```python
from build123d import *

# Parameters (mm, degrees)
BOSS_EXTRUDE1_DEPTH = 10
SKETCH2_R           = 3.829706391
CUT_EXTRUDE1_DEPTH  = 10
CIRPATTERN1_COUNT   = 7
CIRPATTERN1_ANGLE   = 198
CUT_EXTRUDE2_DEPTH  = 10
CIRPATTERN2_COUNT   = 5
CIRPATTERN2_ANGLE   = 60
FILLET1_R           = 3
FILLET2_R           = 1


with BuildPart() as part:
    # Sketch1 → Boss-Extrude1 (new body)
    with BuildSketch(Plane(origin=(0, 0, 0), x_dir=(1, 0, 0), z_dir=(0, 1, 0))):
        with BuildLine():
            Line((-45.667120744, 35.07764347), (41.365145602, 35.07764347))
            ThreePointArc((41.365145602, 35.07764347), (76.442789072, 0), (41.365145602, -35.07764347))
            Line((41.365145602, -35.07764347), (-45.667120744, -35.07764347))
            ThreePointArc((-45.667120744, -35.07764347), (-80.744764215, 0), (-45.667120744, 35.07764347))
        make_face()
    extrude(amount=BOSS_EXTRUDE1_DEPTH)

    # Sketch2 → Cut-Extrude1 (cut)
    with BuildSketch(Plane(origin=(0, 10, 0), x_dir=(1, 0, 0), z_dir=(0, 1, 0))):
        with Locations((0, 21.114814392)):
            Circle(SKETCH2_R)
    cut_extrude1 = extrude(amount=-CUT_EXTRUDE1_DEPTH, mode=Mode.SUBTRACT)

    # CirPattern1: Cut-Extrude1 ×7 about axis
    cirpattern1_axis = Axis((-2.160973251, 0, 0.098022779), (0, 1, 0))
    for i in range(1, CIRPATTERN1_COUNT):
        add(cut_extrude1.rotate(cirpattern1_axis, i * CIRPATTERN1_ANGLE / (CIRPATTERN1_COUNT - 1)), mode=Mode.SUBTRACT)

    # Sketch3 → Cut-Extrude2 (cut)
    with BuildSketch(Plane(origin=(0, 10, 0), x_dir=(1, 0, 0), z_dir=(0, 1, 0))):
        Polygon((36.992565085, 19.326531544), (35.239702282, 24.889438713), (31.298514755, 20.589961412), align=None)
    cut_extrude2 = extrude(amount=-CUT_EXTRUDE2_DEPTH, mode=Mode.SUBTRACT)

    # CirPattern2: Cut-Extrude2 ×5 about axis
    cirpattern2_axis = Axis((-1.883123212, 0, 0.01175113), (0, -1, 0))
    for i in range(1, CIRPATTERN2_COUNT):
        add(cut_extrude2.rotate(cirpattern2_axis, i * CIRPATTERN2_ANGLE / (CIRPATTERN2_COUNT - 1)), mode=Mode.SUBTRACT)

    # Fillet1
    fillet1_edges = [part.edges().sort_by_distance(p)[0] for p in [
        (76.442789072, 10, 0),
        (-2.150987571, 10, -35.07764347),
        (-80.744764215, 10, 0),
        (-2.150987571, 10, 35.07764347),
    ]]
    fillet(fillet1_edges, radius=FILLET1_R)

    # Fillet2
    fillet2_edges = [part.edges().sort_by_distance(p)[0] for p in [
        (-2.150987571, 0, -35.07764347),
        (76.442789072, 0, 0),
        (-2.150987571, 0, 35.07764347),
        (-80.744764215, 0, 0),
    ]]
    fillet(fillet2_edges, radius=FILLET2_R)


solid = part.part
```
The listing builds one solid part. Answer for the finished solid, in the listing's coordinates (mm). Round coordinates to 2 decimals unless told otherwise and drop trailing zeros. Use one line per item in the form item = value. Start each with the question number.
1. The part is cut by section A-A on y = 5.25. Give the number of separate pieces and of enclosed holes in the cut face, then the cut area to 3 significant figures.
2. Consider line 1 (X direction, y = 9, z = -14); line 2 (Z direction, x = -13, y = 8); line 3 (X direction, y = 8, z = -21.5). Determine where each line is inside the solid, lowest interval first. Write a range as [from, to].
3. Given pin 1 Ø7 at (x, z) = (2.34, 20.94) entering from -Y, flat-ended and moving along its own axis, determine where the tip first touches the part or whether it passes through.
4. For a pull along X with two mould halves and no side action, classify faces 1 (the face through (-3, 4, -35.078)), 2 (the face through (40.609, 5.07, 11.276)) as pulls with the +X half, pulls with the -X half, needs draft (parallel to the pull), parting line crosses it, or undercut.
Geometry check:
q1.separate_pieces = 1
q1.enclosed_holes = 12
q1.area = 9,580 mm^2
q2.line_1 = [-76.99, -22.22], [-19.1, 39.74], [40.44, 72.69]
q2.line_2 = [-34.91, -22.54], [-15.2, 18.02], [22.04, 34.91]
q2.line_3 = [-73.17, -14.69], [-9.12, -3.81], [3.81, 32.13], [36.31, 68.86]
q3.pin_1 = through
q4.face_1 = needs draft
q4.face_2 = undercut
